Model file for the job. Use its own axes, mm. Round coordinates to 2 decimals unless told otherwise and drop trailing zeros. Order: outer loops, then holes, each group sorted by start corner. A loop starts at its lowest first (then second) coordinate and runs counter-clockwise, first axis right, second up. Notation, with made-up numbers: (21.25, 47) -> (50.25, 47) arc R20 cw to (50.25, 56) -> close; hole circle Ø10 at (-28, -23). An arc over 180 degrees is marked (long way). Put each result on its own line as item: value. Start each with the question number.
Q1. Cut at A-A, the plane z = 1008. List the corners of the cut face in (x, y), and give its area (3 significant figures).
Q2. Probe L1, parallel to Y at x = -58.5, z = 190; L2, parallel to X at y = 77.5, z = 847.5; L3, parallel to Z at x = -62, y = 54.5. List the from-to ranges inside material, lowest first.
Q3. Flat gauge pins, fed straight in: P1, Ø10, axis at x = -41.61, z = 20, coming from the -Y side; P2, Ø4, axis at x = -35.5, y = 57.5, coming from the -Z side; P3, Ø2.5, axis at x = -64, y = 74, coming from the -Z side; P4, Ø3, axis at x = -60.5, y = 71, coming from the +Z side. Where does each tip first touch, or does it go through?
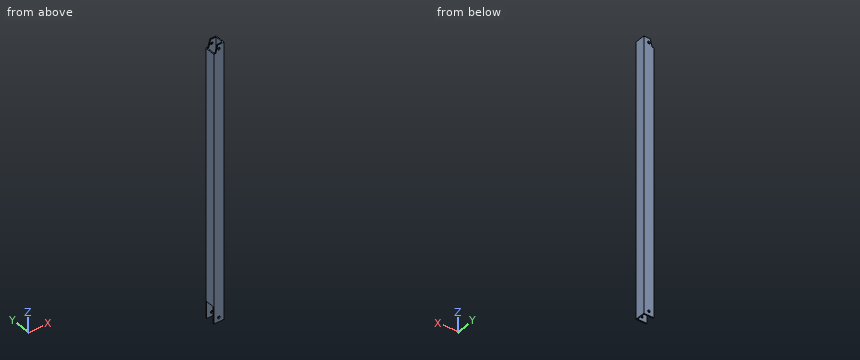
Solid Edge part; units mm, degrees
sketch "Sketch1" plane through (0, 0, 0) normal (0, 0, 1) x (1, 0, 0)
  line L0 (-61.6064, 56.1225) -> (-21.6064, 56.1225)
  line L1 (-21.6064, 56.1225) -> (-21.6064, 96.1225)
  line L2 (-21.6064, 96.1225) -> (-61.6064, 96.1225)
  line L3 (-61.6064, 96.1225) -> (-61.6064, 56.1225)
  line L4 (-66.6064, 51.1225) -> (-16.6064, 51.1225)
  line L5 (-16.6064, 51.1225) -> (-16.6064, 101.1225)
  line L6 (-16.6064, 101.1225) -> (-66.6064, 101.1225)
  line L7 (-66.6064, 101.1225) -> (-66.6064, 51.1225)
  dimension "D1" = 66.6064
  dimension "D2" = 16.6064
  dimension "D3" = 61.6064
extrude "Protrusion1" add sketch "Sketch1" along normal blind 1310
sketch "Sketch2" plane through (-66.6064, 101.1225, 788.35) normal (0, 1, 0) x (0, 0, 1)
  circle A0 centre (501.65, 25) radius 6.1
  circle A1 centre (-768.35, 25) radius 6.1
extrude "Cutout1" cut sketch "Sketch2" against normal through all
sketch "Sketch3" plane through (-66.6064, 81.1225, 788.35) normal (-1, 0, 0) x (0, 0, 1)
  line L0 (-788.35, 15) -> (-788.35, -25)
  line L1 (-788.35, -25) -> (-788.34, -25)
  line L2 (-788.34, -25) -> (-788.34, 15)
  line L3 (-788.34, 15) -> (-788.35, 15)
  dimension "D1" = 788.34
  dimension "D2" = 788.34
extrude "Cutout2" cut sketch "Sketch3" against normal blind 5
sketch "Sketch4" plane through (-16.6064, 81.1225, 788.35) normal (1, 0, 0) x (0, 0, 1)
  line L0 (-788.35, -15) -> (-788.34, -15)
  line L1 (-788.34, -15) -> (-788.34, 25)
  line L2 (-788.34, 25) -> (-788.35, 25)
  line L3 (-788.35, 25) -> (-788.35, -15)
  dimension "D1" = 788.34
  dimension "D2" = 788.34
extrude "ExtrudedCutout_3" cut sketch "Sketch4" against normal blind 5
sketch "Sketch5" plane through (-66.6064, 51.1225, 704.15) normal (0, -1, 0) x (0, 0, -1)
  line L0 (-605.85, 0) -> (-605.85, 19.3782)
  line L1 (-570.85, 10) -> (-605.85, 19.3782)
  line L2 (-570.85, 10) -> (-570.85, 0)
  line L3 (-570.85, 0) -> (-605.85, 0)
  dimension "D1" = 570.85
  dimension "D2" = 570.85
extrude "Cutout3" cut sketch "Sketch5" against normal through all
sketch "Sketch6" plane through (-66.6064, 76.1225, 637.5) normal (-1, 0, 0) x (0, 0, 1)
  line L0 (-637.49, -20) -> (-557.49, -20)
  line L1 (-557.49, -20) -> (-557.49, 20)
  line L2 (-557.49, 20) -> (-637.49, 20)
  line L3 (-637.49, 20) -> (-637.49, -20)
  dimension "D1" = 637.49
  dimension "D2" = 557.49
extrude "Cutout4" cut sketch "Sketch6" against normal up to next
properties material "Aluminum, 6061-T6"
Ans:
1. outline: (-66.61, 51.12) -> (-16.61, 51.12) -> (-16.61, 101.12) -> (-66.61, 101.12) -> close; hole (-61.61, 56.12) -> (-21.61, 56.12) -> (-21.61, 96.12) -> (-61.61, 96.12) -> close
1. area: 900 mm^2
2. L1: y = 51.12 to 56.12, 96.12 to 101.12
2. L2: x = -66.61 to -61.61, -21.61 to -16.61
2. L3: z = 0 to 1275
3. P1: passes through
3. P2: stops at z = 0
3. P3: stops at z = 80.01
3. P4: stops at z = 1275
